from build123d import *

# Parameters (mm, degrees)
F0_W      = 203.2
F0_H      = 127
F1_DEPTH  = 127
F3_DEPTH  = 76.2
F4_SIZE2  = 101.6
F4_SIZE   = 76.2
F5_R      = 5.08
F6_R      = 15.24
F7_DEPTH  = 50.801
F8_R      = 15.24
F10_DEPTH = 127.001


with BuildPart() as f1:
    # F0 (on Front) → F1 (new body)
    with BuildSketch(Plane.XZ):
        with Locations((2.8009600937, 11.9344207702)):
            Rectangle(F0_W, F0_H)
    extrude(amount=F1_DEPTH)

    # F2 (on face) → F3 (cut)
    with BuildSketch(Plane.XZ.offset(127)):
        Polygon((-35.2990399063, 11.9344207702), (-35.2990399063, -51.5655792298), (104.4009600937, -51.5655792298), (104.4009600937, 75.4344207702), (2.8009600937, 75.4344207702), (2.8009600937, 11.9344207702), align=None)
    extrude(amount=-F3_DEPTH, mode=Mode.SUBTRACT)

    # F4
    f4_edges = [f1.edges().sort_by_distance(p)[0] for p in [
        (104.40096, -25.4, 75.434421),
    ]]
    f4_side = f1.faces().sort_by_distance((-18.970468, -52.614286, 75.434421))[0]
    chamfer(f4_edges, length=F4_SIZE, length2=F4_SIZE2, reference=f4_side)

    # F5
    f5_edges = [f1.edges().sort_by_distance(p)[0] for p in [
        (-47.99904, -127, 75.434421),
        (-98.79904, -63.5, 75.434421),
        (-35.29904, 0, 75.434421),
        (2.80096, -88.9, 75.434421),
        (15.50096, -50.8, 75.434421),
        (2.80096, -50.8, 43.684421),
        (2.80096, -127, 43.684421),
        (2.80096, -88.9, 11.934421),
        (-35.29904, -50.8, -19.815579),
        (34.55096, -50.8, -51.565579),
        (-35.29904, -88.9, -51.565579),
        (-35.29904, -127, -19.815579),
        (-67.04904, -127, -51.565579),
        (-98.79904, -127, 11.934421),
        (2.80096, 0, -51.565579),
        (-98.79904, 0, 11.934421),
        (-98.79904, -63.5, -51.565579),
        (28.20096, -25.4, 75.434421),
        (-16.24904, -127, 11.934421),
        (-16.24904, -50.8, 11.934421),
    ]]
    fillet(f5_edges, radius=F5_R)

    # F6 (on face) → F7 (cut, through all)
    with BuildSketch(Plane.XZ.offset(50.8)):
        with Locations((20.5809600937, -5.8455792298)):
            Circle(F6_R)
    extrude(amount=-F7_DEPTH, mode=Mode.SUBTRACT)

    # F8 (on face) → F10 (cut, through all)
    with BuildSketch(Plane.XY.offset(75.4344207702)):
        with Locations((-74.706427753, -81.28)):
            Circle(F8_R)
    extrude(amount=-F10_DEPTH, mode=Mode.SUBTRACT)


solid = f1.part
Geometry: final body of the model. Coordinates: model frame, mm. A direction names the side the tool comes from. Give positions to 0.01 mm unless a question says otherwise; leave off trailing zeros. Order: outer loops, then holes, each group sorted by start corner. A loop starts at its lowest first (then second) coordinate and runs counter-clockwise, first axis right, second up. Notation, with made-up numbers: (72.25, 63.5) -> (115.25, 63.5) arc R23 ccw to (115.25, 81.5) -> close; hole circle Ø10 at (-10.75, 4). An arc over 180 degrees is marked (long way). Put each result on its own line as item: value.
Q1. Section B-B, the plane y = -81.28. Return loops of the section in (x, z).
Here are the results:
outline: (-98.8, -46.49) arc R5.08 ccw to (-93.72, -51.57) -> (-89.95, -51.57) -> (-89.95, 75.43) -> (-93.72, 75.43) arc R5.08 ccw to (-98.8, 70.35) -> close; (-59.47, -51.57) -> (-40.38, -51.57) arc R5.08 ccw to (-35.3, -46.49) -> (-35.3, 11.93) -> (-2.28, 11.93) arc R5.08 ccw to (2.8, 17.01) -> (2.8, 70.35) arc R5.08 ccw to (-2.28, 75.43) -> (-59.47, 75.43) -> close
Q2. Section D-D, the plane y = -107. Return loops of the section in (x, z).
Here are the results:
outline: (-98.8, -46.49) arc R5.08 ccw to (-93.72, -51.57) -> (-40.38, -51.57) arc R5.08 ccw to (-35.3, -46.49) -> (-35.3, 11.93) -> (-2.28, 11.93) arc R5.08 ccw to (2.8, 17.01) -> (2.8, 70.35) arc R5.08 ccw to (-2.28, 75.43) -> (-93.72, 75.43) arc R5.08 ccw to (-98.8, 70.35) -> close
Q3. Reachability of faces 1 (the face through (-97.27, -1.45, 12.75)), 2 (the face through (-21.6, -125.55, 13.46)) from +Z, -Z, +X, -X, +Y, -Y: full face, straight path, thin tool, end or side. Return the list, or none.
Here are the results:
face 1: +Z, -Z, -X, +Y
face 2: -Z, +X, -Y
Q4. Section A-A, the plane z = -31. Return loops of the section in (x, y).
Here are the results:
outline: (-98.8, -121.92) arc R5.08 ccw to (-93.72, -127) -> (-40.38, -127) arc R5.08 ccw to (-35.3, -121.92) -> (-35.3, -55.88) arc R5.08 cw to (-30.22, -50.8) -> (104.4, -50.8) -> (104.4, 0) -> (-93.72, 0) arc R5.08 ccw to (-98.8, -5.08) -> close; hole circle Ø30.48 at (-74.71, -81.28)
Q5. Material intervals for L1, parallel to Y at x = 63, z = -13; L2, parallel to X at y = -106, z = 63.5; L3, parallel to X at y = -81, z = -11, sorted ascending.
Here are the results:
L1: y = -50.8 to 0
L2: x = -98.8 to 2.8
L3: x = -98.8 to -89.94, -59.47 to -35.3
Q6. Pin query (flat end, axial travel): pin 1 (10 mm diameter, centred on x = -4, y = -72.5, fed in from -Z); pin 2 (5 mm diameter, centred on x = 41, z = 7.5, fed in from -Y); pin 3 (4 mm diameter, centred on y = -37.5, z = -21.5, fed in from +X). Return the tip coordinate at first contact, or that it passes through.
Here are the results:
pin 1: stops at z = 11.93
pin 2: stops at y = -50.8
pin 3: stops at x = 102.4
Q7. Draft query along Y for faces 3 (the face through (-18, 0, 13)), 4 (the face through (-18, -37, -51.566)), 5 (the face through (38.03, -49.35, -50.04)), 6 (the face through (-60.63, -87.12, 12.82)). Return one class per face: released by +Y, released by -Y, zero draft, split by the parting line, or undercut.
Here are the results:
face 3: released by +Y
face 4: zero draft
face 5: released by -Y
face 6: undercut
Q8. Section C-C, the plane z = -3. Return loops of the section in (x, y).
Here are the results:
outline: (-98.8, -121.92) arc R5.08 ccw to (-93.72, -127) -> (-40.38, -127) arc R5.08 ccw to (-35.3, -121.92) -> (-35.3, -55.88) arc R5.08 cw to (-30.22, -50.8) -> (5.61, -50.8) -> (5.61, 0) -> (-93.72, 0) arc R5.08 ccw to (-98.8, -5.08) -> close; (35.55, -50.8) -> (87.03, -50.8) -> (87.03, 0) -> (35.55, 0) -> close; hole circle Ø30.48 at (-74.71, -81.28)
